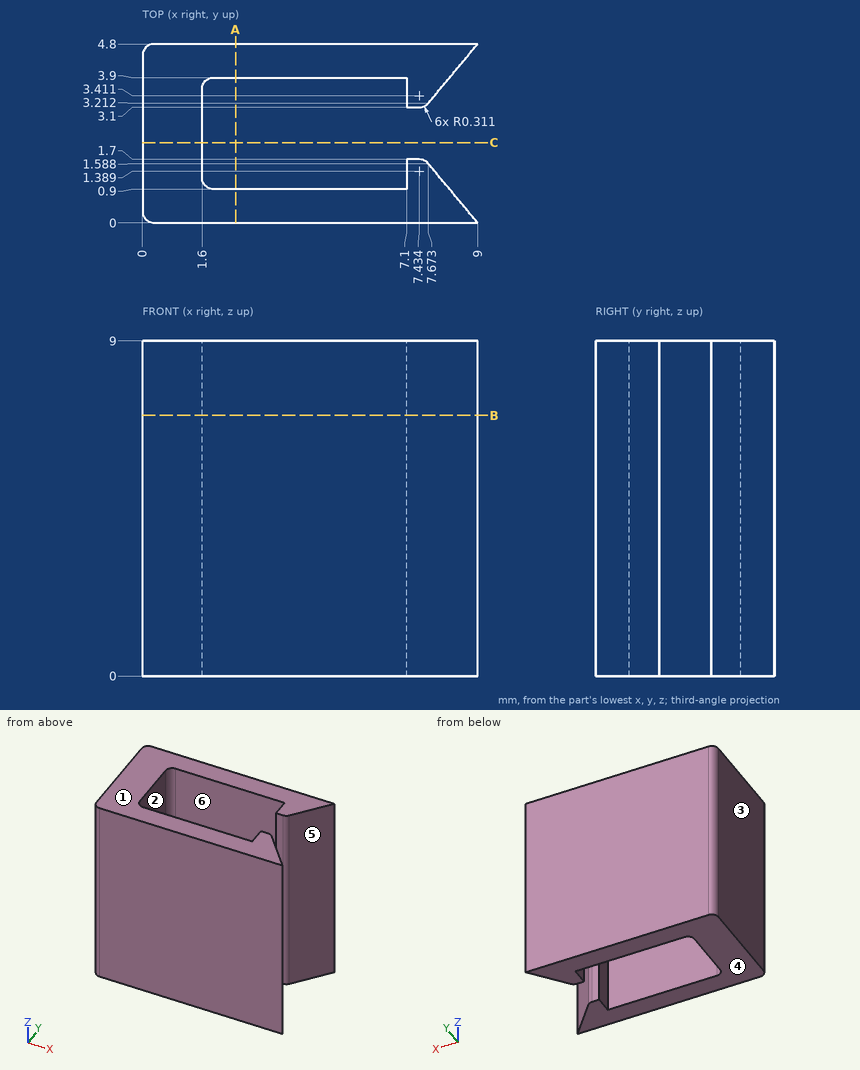
Input: dimensioned drawing with shaded views. Units: mm. Origin: part minimum x, y, z. A direction names the side the tool comes from. Coordinates: 2 decimals unless noted, no trailing zeros. Order: outer loops, then holes, each group sorted by start corner. A loop starts at its lowest first (then second) coordinate and runs counter-clockwise, first axis right, second up. Notation, with made-up numbers: (16.5, -14) - (64.5, -14) arc R22 cw to (64.5, 7) - close; hole circle Ø1 at (32, 70.25). An arc over 180 degrees is marked (long way). Return JSON: item names as keys, results as strings. Group by question number.
1. Cut plane B-B (z = 7). Output: boundary loops of the cut face in (x, y).
2. Cut plane C-C (y = 2.15). Output: boundary loops of the cut face in (x, z).
3. Material intervals for line 1 along Y through (x, z) = (6.25, 2.75); line 2 along X through (y, z) = (2.7, 3.5); line 3 along X through (y, z) = (3.3, 2.5) (1 decimal), sorted ascending. Write a range as [from, to].
4. Cut plane A-A (x = 2.5). Output: boundary loops of the cut face in (y, z), plus the area to 3 significant figures.
5. Pull-direction query (X, two-part tool) for the marked faces 1, 2 and 3; classes: pulls with the +X half, pulls with the -X half, needs draft (parallel to the pull), parting line crosses it, or undercut.
6. Set-up query: the marked faces 4, 5 and 6. Return all of +Z, -Z, +X, -X, +Y, -Y with unobstructed straight access to the full face (end or side cutting, diameter ignored); none if empty.
7. Pin query (flat end, axial travel): pin 1 (1 mm diameter, centred on y = 3.5, z = 3, fed in from +X); pin 2 (1 mm diameter, centred on y = 2.5, z = 6.5, fed in from +X). Return the tip coordinate at first contact, or that it passes through.
Resolved:
{
 "1": {"outline": "(0, 0.31) arc R0.31 ccw to (0.31, 0) - (9, 0) - (7.67, 1.59) arc R0.31 ccw to (7.43, 1.7) - (7.1, 1.7) - (7.1, 0.9) - (1.91, 0.9) arc R0.31 cw to (1.6, 1.21) - (1.6, 3.59) arc R0.31 cw to (1.91, 3.9) - (7.1, 3.9) - (7.1, 3.1) - (7.43, 3.1) arc R0.31 ccw to (7.67, 3.21) - (9, 4.8) - (0.31, 4.8) arc R0.31 ccw to (0, 4.49) - close"},
 "2": {"outline": "(0, 0) - (1.6, 0) - (1.6, 9) - (0, 9) - close"},
 "3": {"line 1": "y = [0, 0.9], [3.9, 4.8]", "line 2": "x = [0, 1.6]", "line 3": "x = [0, 1.6], [7.1, 7.7]"},
 "4": {"outline": "(0, 0) - (0.9, 0) - (0.9, 9) - (0, 9) - close; (3.9, 0) - (4.8, 0) - (4.8, 9) - (3.9, 9) - close", "area": "16.2 mm²"},
 "5": {"face 1": "needs draft", "face 2": "undercut", "face 3": "pulls with the -X half"},
 "6": {"face 4": "-Z, +X, -X, +Y, -Y", "face 5": "+Z, -Z, +X", "face 6": "+Z, -Z"},
 "7": {"pin 1": "stops at x = 8.33", "pin 2": "stops at x = 1.6"}
}
